CAD build for the part. Positions are in the model's coordinates, mm. Face numbers are marked on the shaded views. Coordinates: 2 decimals unless noted, no trailing zeros. Loops run counter-clockwise (first coordinate to the right, second up) from the corner with the lowest first, then second, coordinate; pieces in that order, holes last. Notation, with made-up numbers: (12, 56) -> (50, 56) arc R11 cw to (50, 74) -> close; hole circle Ø9 at (35.5, 26.25). An arc over 180 degrees is marked (long way). Write each question's results on one line, items separated by ' | '.
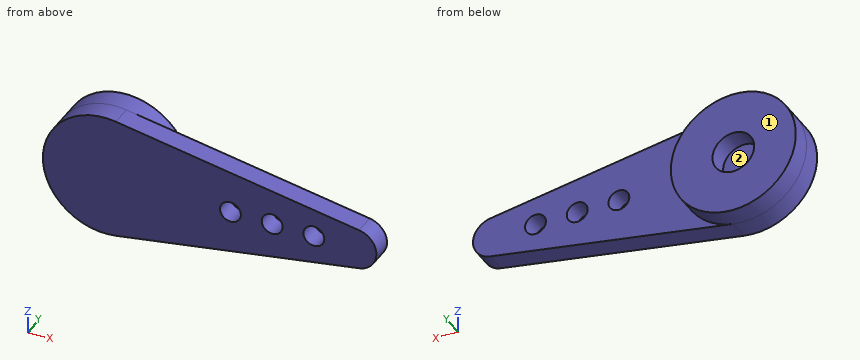
```python
from build123d import *
from build123d.topology import SkipClean

# Parameters (mm, degrees)
BOSS_EXTRUDE1_DEPTH = 5
SKETCH2_R           = 15
BOSS_EXTRUDE2_DEPTH = 5
SKETCH3_R           = 5
CUT_EXTRUDE1_DEPTH  = 5
SKETCH4_R           = 2.5
CUT_EXTRUDE2_DEPTH  = 5


with BuildPart() as part:
    # Sketch1 → Boss-Extrude1 (new body)
    with BuildSketch(Plane(origin=(0, 0, 0), x_dir=(1, 0, 0), z_dir=(0, 1, 0))):
        with BuildLine():
            Line((2.5, 14.790199458), (60.833333333, 4.930066486))
            ThreePointArc((60.833333333, 4.930066486), (65, 0), (60.833333333, -4.930066486))
            Line((60.833333333, -4.930066486), (2.5, -14.790199458))
            ThreePointArc((2.5, -14.790199458), (-15, 0), (2.5, 14.790199458))
        make_face()
    extrude(amount=BOSS_EXTRUDE1_DEPTH)

    # Sketch2 → Boss-Extrude2 (add)
    with SkipClean():  # the faces are left unmerged after this step: merging them gives an invalid solid
        with BuildSketch(Plane(origin=(0, 5, 0), x_dir=(1, 0, 0), z_dir=(0, 1, 0))):
            with Locations(Location((0, 0, 0), (0, 0, 80.405931773))):
                Circle(SKETCH2_R)
        extrude(amount=BOSS_EXTRUDE2_DEPTH)

    # Sketch3 → Cut-Extrude1 (cut)
    with SkipClean():  # the faces are left unmerged after this step: merging them gives an invalid solid
        with BuildSketch(Plane(origin=(0, 10, 0), x_dir=(1, 0, 0), z_dir=(0, 1, 0))):
            with Locations(Location((0, 0, 0), (0, 0, 270))):
                Circle(SKETCH3_R)
        extrude(amount=-CUT_EXTRUDE1_DEPTH, mode=Mode.SUBTRACT)

    # Sketch4 → Cut-Extrude2 (cut)
    with SkipClean():  # the faces are left unmerged after this step: merging them gives an invalid solid
        with BuildSketch(Plane(origin=(0, 5, 0), x_dir=(1, 0, 0), z_dir=(0, 1, 0))):
            with Locations(Location((50, 0, 0), (0, 0, 270))):
                Circle(SKETCH4_R)
            with Locations(Location((40, 0, 0), (0, 0, 270))):
                Circle(SKETCH4_R)
            with Locations(Location((30, 0, 0), (0, 0, 270))):
                Circle(SKETCH4_R)
        extrude(amount=-CUT_EXTRUDE2_DEPTH, mode=Mode.SUBTRACT)


solid = part.part
```
Q1. Cut at A-A on z = 0. Write the cut outline in (x, y), and give its area (3 significant figures).
Results are:
outline: (-15, 0) -> (27.5, 0) -> (27.5, 5) -> (15, 5) -> (15, 10) -> (5, 10) -> (5, 5) -> (-5, 5) -> (-5, 10) -> (-15, 10) -> close; (32.5, 0) -> (37.5, 0) -> (37.5, 5) -> (32.5, 5) -> close; (42.5, 0) -> (47.5, 0) -> (47.5, 5) -> (42.5, 5) -> close; (52.5, 0) -> (65, 0) -> (65, 5) -> (52.5, 5) -> close | area: 425 mm^2
Q2. Cut at D-D on x = 0. Write the cut outline in (y, z), and give its area (3 significant figures).
Results are:
outline: (0, -15) -> (10, -15) -> (10, -5) -> (5, -5) -> (5, 5) -> (10, 5) -> (10, 15) -> (0, 15) -> close | area: 250 mm^2
Q3. Drop flat-ended pins along their axis: pin 1 (5 mm diameter, centred on x = -1.5, z = 1.5, fed in from +Y); pin 2 (6 mm diameter, centred on y = 6, z = 1, fed in from -X); pin 3 (6 mm diameter, centred on y = 1.5, z = -4.5, fed in from -X); pin 4 (3 mm diameter, centred on x = 30, z = 0, fed in from -Y). Give the stop position or say it passes through.
Results are:
pin 1: y = 5 | pin 2: x = -15 | pin 3: x = -14.92 | pin 4: through
Q4. Wall check: L1, parallel to Y at x = 21, z = -11; L2, parallel to X at y = 7.75, z = 0; L3, parallel to Z at x = 0.5, y = 1.25. Give the ranges that are in metal, low to high. Write a range as from..to.
Results are:
L1: 0..5 | L2: -15..-5, 5..15 | L3: -14.99..14.99
Q5. Cut at B-B on x = 50. Write the cut outline in (y, z).
Results are:
outline: (0, -6.76) -> (5, -6.76) -> (5, -2.5) -> (0, -2.5) -> close; (0, 2.5) -> (5, 2.5) -> (5, 6.76) -> (0, 6.76) -> close
Q6. Cut at C-C on y = 1. Write the cut outline in (x, z).
Results are:
outline: (2.5, -14.79) -> (60.83, -4.93) arc R5 ccw to (60.83, 4.93) -> (2.5, 14.79) arc R15 ccw (long way) to start; hole circle Ø5 at (30, 0); hole circle Ø5 at (40, 0); hole circle Ø5 at (50, 0)
Q7. Pull direction Z, two halves, no side cores. Call the marked faces 1 and 2: +Z half, -Z half, draft (parallel to the pull), parting line (faces both ways), or undercut.
Results are:
face 1: draft | face 2: undercut
